from build123d import *

# Parameters (mm, degrees)
SKETCH1_R           = 29.5
SKETCH1_R_2         = 27.5
BOSS_EXTRUDE2_DEPTH = 14
SKETCH3_R           = 29.5
SKETCH3_R_2         = 1.5
BOSS_EXTRUDE3_DEPTH = 5
CHAMFER1_SIZE       = 3
CHAMFER1_SIZE2      = 17.013845459
FILLET1_R           = 2
SKETCH4_R           = 2
BOSS_EXTRUDE4_DEPTH = 5.4
CHAMFER2_SIZE       = 0.2


with BuildPart() as part:
    # Sketch1 → Boss-Extrude2 (new body)
    with BuildSketch(Plane(origin=(0, 0, 0), x_dir=(1, 0, 0), z_dir=(0, 1, 0))):
        with Locations(Location((0, 0, 0), (0, 0, 270))):
            Circle(SKETCH1_R)
        with Locations(Location((0, 0, 0), (0, 0, 270))):
            Circle(SKETCH1_R_2, mode=Mode.SUBTRACT)
    extrude(amount=BOSS_EXTRUDE2_DEPTH)

    # Sketch3 → Boss-Extrude3 (add)
    with BuildSketch(Plane(origin=(0, 14, 0), x_dir=(1, 0, 0), z_dir=(0, 1, 0))):
        with Locations(Location((0, 0, 0), (0, 0, 270))):
            Circle(SKETCH3_R)
        with Locations(Location((0, 6, 0), (0, 0, 270))):
            Circle(SKETCH3_R_2, mode=Mode.SUBTRACT)
        with Locations(Location((6, 0, 0), (0, 0, 270))):
            Circle(SKETCH3_R_2, mode=Mode.SUBTRACT)
        with Locations(Location((0, -6, 0), (0, 0, 270))):
            Circle(SKETCH3_R_2, mode=Mode.SUBTRACT)
        with Locations(Location((-6, 0, 0), (0, 0, 270))):
            Circle(SKETCH3_R_2, mode=Mode.SUBTRACT)
    extrude(amount=BOSS_EXTRUDE3_DEPTH)

    # Chamfer1
    chamfer1_edges = [part.edges().sort_by_distance(p)[0] for p in [
        (0, 19, -29.5),
    ]]
    chamfer1_side = [part.faces().sort_by_distance(p)[0] for p in [
        (0, 9.5, -29.5),
    ]]
    chamfer(chamfer1_edges, length=CHAMFER1_SIZE, length2=CHAMFER1_SIZE2, reference=chamfer1_side[0])

    # Fillet1
    fillet1_edges = [part.edges().sort_by_distance(p)[0] for p in [
        (0, 16, -29.5),
    ]]
    fillet(fillet1_edges, radius=FILLET1_R)

    # Sketch4 → Boss-Extrude4 (add)
    with BuildSketch(Plane(origin=(0, 19, 0), x_dir=(1, 0, 0), z_dir=(0, 1, 0))):
        with Locations(Location((0, 0, 0), (0, 0, 90))):
            Circle(SKETCH4_R)
    extrude(amount=BOSS_EXTRUDE4_DEPTH)

    # Chamfer2
    chamfer2_edges = [part.edges().sort_by_distance(p)[0] for p in [
        (0, 24.4, 2),
    ]]
    chamfer(chamfer2_edges, length=CHAMFER2_SIZE)


solid = part.part
Geometry: final body of the model. Coordinates: model frame, mm. Give positions to 0.01 mm unless a question says otherwise; leave off trailing zeros. Order: outer loops, then holes, each group sorted by start corner. A loop starts at its lowest first (then second) coordinate and runs counter-clockwise, first axis right, second up. Notation, with made-up numbers: (-21.75, 4.5) -> (24.25, 4.5) arc R18 ccw to (24.25, 28.5) -> close; hole circle Ø3 at (9.25, 82). An arc over 180 degrees is marked (long way). Answer as a JSON object with one key per item and string values.
Q1. Draft query along X for faces 1 (the cylindrical face through (-24.397, 6.902, 12.69)), 2 (the flat face through (-20, 0, 20)), 3 (the flat face through (0, 14, 0)), 4 (the cylindrical face through (2, 22, 0)). Return one class per face: released by +X, released by -X, zero draft, split by the parting line, or undercut.
Entries:
{"face 1": "undercut", "face 2": "zero draft", "face 3": "undercut", "face 4": "split by the parting line"}
Q2. First-contact query: pin 1 (1 mm diameter, centred on x = 18, y = 6, fed in from +Z); pin 2 (6 mm diameter, centred on x = 4, z = -16.5, fed in from +Y); pin 3 (2.5 mm diameter, centred on x = 0, z = 6, fed in from -Y); pin 4 (10 mm diameter, centred on x = 12, z = 22, fed in from -Y). Flat tips, straight axial feed; report the tip coordinate or a pass-through.
Entries:
{"pin 1": "stops at z = 23.75", "pin 2": "stops at y = 18.74", "pin 3": "passes through", "pin 4": "stops at y = 0"}
Q3. Material intervals for probe 1 along X at (y, z) = (8.5, 0); probe 2 along Y at (x, z) = (0, 10); probe 3 along Z at (x, y) = (7.5, 12.5), sorted ascending.
Entries:
{"probe 1": "x = -29.5 to -27.5, 27.5 to 29.5", "probe 2": "y = 14 to 19", "probe 3": "z = -28.53 to -26.46, 26.46 to 28.53"}
Q4. Section B-B (y = 12.25). Output: boundary loops of the cut face in (x, z).
Entries:
{"outline": "circle Ø59 at (0, 0); hole circle Ø55 at (0, 0)"}
Q5. Section A-A (x = 0). State how many separate pieces and enclosed holes the cut face has, plus the area to 3 significant figures.
Entries:
{"separate pieces": "3", "enclosed holes": "0", "area": "290 mm^2"}
Q6. Section C-C (y = 20). Output: boundary loops of the cut face in (x, z), plus the area to 3 significant figures.
Entries:
{"outline": "circle Ø4 at (0, 0)", "area": "12.6 mm^2"}
